```python
from build123d import *

# Parameters (mm, degrees)
SKETCH1_R           = 27
SKETCH1_R_2         = 1
SKETCH1_W           = 2
SKETCH1_H           = 6
SKETCH1_W_2         = 6
SKETCH1_H_2         = 2
BOSS_EXTRUDE1_DEPTH = 2


with BuildPart() as part:
    # Sketch1 → Boss-Extrude1 (new body)
    with BuildSketch(Plane.XY):
        with BuildLine():
            Line((23, 35), (35, 23))
            Line((35, 23), (35, 19))
            ThreePointArc((35, 19), (31, 0), (35, -19))
            Line((35, -19), (35, -23))
            Line((35, -23), (23, -35))
            Line((23, -35), (19, -35))
            ThreePointArc((19, -35), (0, -31), (-19, -35))
            Line((-19, -35), (-23, -35))
            Line((-23, -35), (-35, -23))
            Line((-35, -23), (-35, -19))
            ThreePointArc((-35, -19), (-31, 0), (-35, 19))
            Line((-35, 19), (-35, 23))
            Line((-35, 23), (-23, 35))
            Line((-23, 35), (-19, 35))
            ThreePointArc((-19, 35), (0, 31), (19, 35))
            Line((19, 35), (23, 35))
        make_face()
        Circle(SKETCH1_R, mode=Mode.SUBTRACT)
        with Locations((26, 26)):
            Circle(SKETCH1_R_2, mode=Mode.SUBTRACT)
        with Locations((21, 21)):
            Circle(SKETCH1_R_2, mode=Mode.SUBTRACT)
        with Locations((26, -26)):
            Circle(SKETCH1_R_2, mode=Mode.SUBTRACT)
        with Locations((-26, -26)):
            Circle(SKETCH1_R_2, mode=Mode.SUBTRACT)
        with Locations((-26, 26)):
            Circle(SKETCH1_R_2, mode=Mode.SUBTRACT)
        with BuildLine():
            Line((18, 30.970831308), (18, 24.718414189))
            ThreePointArc((18, 24.718414189), (17.465474668, 23.833352985), (16.433333333, 23.894467049))
            ThreePointArc((16.433333333, 23.894467049), (12.522883391, 26.15678481), (8.308523463, 27.78432))
            ThreePointArc((8.308523463, 27.78432), (7.59677162, 28.801490124), (8.423552466, 29.727589027))
            ThreePointArc((8.423552466, 29.727589027), (12.589647358, 30.640619364), (16.66084788, 31.911562853))
            ThreePointArc((16.66084788, 31.911562853), (17.574825139, 31.789107582), (18, 30.970831308))
        make_face(mode=Mode.SUBTRACT)
        with BuildLine():
            Line((-18, 30.970831308), (-18, 24.718414189))
            ThreePointArc((-18, 24.718414189), (-17.465474668, 23.833352985), (-16.433333333, 23.894467049))
            ThreePointArc((-16.433333333, 23.894467049), (-12.522883391, 26.156784809), (-8.308523463, 27.78432))
            ThreePointArc((-8.308523463, 27.78432), (-7.59677162, 28.801490124), (-8.423552466, 29.727589027))
            ThreePointArc((-8.423552466, 29.727589027), (-12.589647358, 30.640619364), (-16.66084788, 31.911562853))
            ThreePointArc((-16.66084788, 31.911562853), (-17.574825139, 31.789107582), (-18, 30.970831308))
        make_face(mode=Mode.SUBTRACT)
        with Locations((-21, 29)):
            Rectangle(SKETCH1_W, SKETCH1_H, mode=Mode.SUBTRACT)
        with Locations((21, 29)):
            Rectangle(SKETCH1_W, SKETCH1_H, mode=Mode.SUBTRACT)
        with Locations((29, 21)):
            Rectangle(SKETCH1_W_2, SKETCH1_H_2, mode=Mode.SUBTRACT)
        with Locations((29, -21)):
            Rectangle(SKETCH1_W_2, SKETCH1_H_2, mode=Mode.SUBTRACT)
        with BuildLine():
            Line((30.970831308, 18), (24.718414189, 18))
            ThreePointArc((24.718414189, 18), (23.833352985, 17.465474668), (23.894467049, 16.433333333))
            ThreePointArc((23.894467049, 16.433333333), (26.156784809, 12.522883391), (27.78432, 8.308523463))
            ThreePointArc((27.78432, 8.308523463), (28.801490124, 7.59677162), (29.727589027, 8.423552466))
            ThreePointArc((29.727589027, 8.423552466), (30.640619364, 12.589647358), (31.911562853, 16.66084788))
            ThreePointArc((31.911562853, 16.66084788), (31.789107582, 17.574825139), (30.970831308, 18))
        make_face(mode=Mode.SUBTRACT)
        with BuildLine():
            Line((30.970831308, -18), (24.718414189, -18))
            ThreePointArc((24.718414189, -18), (23.833352985, -17.465474668), (23.894467049, -16.433333333))
            ThreePointArc((23.894467049, -16.433333333), (26.15678481, -12.522883391), (27.78432, -8.308523463))
            ThreePointArc((27.78432, -8.308523463), (28.801490124, -7.59677162), (29.727589027, -8.423552466))
            ThreePointArc((29.727589027, -8.423552466), (30.640619364, -12.589647358), (31.911562853, -16.66084788))
            ThreePointArc((31.911562853, -16.66084788), (31.789107582, -17.574825139), (30.970831308, -18))
        make_face(mode=Mode.SUBTRACT)
        with Locations((21, -29)):
            Rectangle(SKETCH1_W, SKETCH1_H, mode=Mode.SUBTRACT)
        with Locations((-21, -29)):
            Rectangle(SKETCH1_W, SKETCH1_H, mode=Mode.SUBTRACT)
        with BuildLine():
            Line((18, -30.970831308), (18, -24.718414189))
            ThreePointArc((18, -24.718414189), (17.465474668, -23.833352985), (16.433333333, -23.894467049))
            ThreePointArc((16.433333333, -23.894467049), (12.522883391, -26.156784809), (8.308523463, -27.78432))
            ThreePointArc((8.308523463, -27.78432), (7.59677162, -28.801490124), (8.423552466, -29.727589027))
            ThreePointArc((8.423552466, -29.727589027), (12.589647358, -30.640619364), (16.66084788, -31.911562853))
            ThreePointArc((16.66084788, -31.911562853), (17.574825139, -31.789107582), (18, -30.970831308))
        make_face(mode=Mode.SUBTRACT)
        with BuildLine():
            Line((-18, -30.970831308), (-18, -24.718414189))
            ThreePointArc((-18, -24.718414189), (-17.465474668, -23.833352985), (-16.433333333, -23.894467049))
            ThreePointArc((-16.433333333, -23.894467049), (-12.522883391, -26.15678481), (-8.308523463, -27.78432))
            ThreePointArc((-8.308523463, -27.78432), (-7.59677162, -28.801490124), (-8.423552466, -29.727589027))
            ThreePointArc((-8.423552466, -29.727589027), (-12.589647358, -30.640619364), (-16.66084788, -31.911562853))
            ThreePointArc((-16.66084788, -31.911562853), (-17.574825139, -31.789107582), (-18, -30.970831308))
        make_face(mode=Mode.SUBTRACT)
        with Locations((-29, -21)):
            Rectangle(SKETCH1_W_2, SKETCH1_H_2, mode=Mode.SUBTRACT)
        with Locations((-29, 21)):
            Rectangle(SKETCH1_W_2, SKETCH1_H_2, mode=Mode.SUBTRACT)
        with BuildLine():
            Line((-30.970831308, -18), (-24.718414189, -18))
            ThreePointArc((-24.718414189, -18), (-23.833352985, -17.465474668), (-23.894467049, -16.433333333))
            ThreePointArc((-23.894467049, -16.433333333), (-26.156784809, -12.522883391), (-27.78432, -8.308523463))
            ThreePointArc((-27.78432, -8.308523463), (-28.801490124, -7.59677162), (-29.727589027, -8.423552466))
            ThreePointArc((-29.727589027, -8.423552466), (-30.640619364, -12.589647358), (-31.911562853, -16.66084788))
            ThreePointArc((-31.911562853, -16.66084788), (-31.789107582, -17.574825139), (-30.970831308, -18))
        make_face(mode=Mode.SUBTRACT)
        with BuildLine():
            Line((-30.970831308, 18), (-24.718414189, 18))
            ThreePointArc((-24.718414189, 18), (-23.833352985, 17.465474668), (-23.894467049, 16.433333333))
            ThreePointArc((-23.894467049, 16.433333333), (-26.15678481, 12.522883391), (-27.78432, 8.308523463))
            ThreePointArc((-27.78432, 8.308523463), (-28.801490124, 7.59677162), (-29.727589027, 8.423552466))
            ThreePointArc((-29.727589027, 8.423552466), (-30.640619364, 12.589647358), (-31.911562853, 16.66084788))
            ThreePointArc((-31.911562853, 16.66084788), (-31.789107582, 17.574825139), (-30.970831308, 18))
        make_face(mode=Mode.SUBTRACT)
    extrude(amount=BOSS_EXTRUDE1_DEPTH)


solid = part.part
```
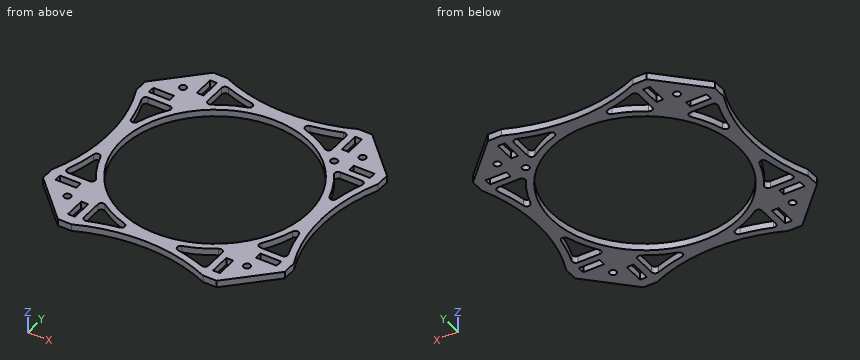
Part model, mm, in its own coordinate system. Round coordinates to 2 decimals unless told otherwise and drop trailing zeros. Order: outer loops, then holes, each group sorted by start corner. A loop starts at its lowest first (then second) coordinate and runs counter-clockwise, first axis right, second up. Notation, with made-up numbers: M 4,72.5 L 39,72.5 A23 ccw 39,109.5 Z; hole C 55.25,-34.75 d1. An arc over 180 degrees is marked long. Answer in a Markdown table with one row per item. Add a question column.
Q1. Wall check: L1, parallel to X at y = -29, z = 1.65; L2, parallel to X at y = -1, z = 1.6; L3, parallel to X at y = -11, z = 0.95. Give the ranges that are in metal, low to high. Write a range as from..to.
Q2. Cut at A-A on x = 0. Give the cut face in (y, z).
Q3. Pin check, flat tips, straight feed: pin 1 (0.6 mm diameter, centred on y = 29.5, z = 0.5, fed in from -X); pin 2 (0.6 mm diameter, centred on y = -28, z = 1, fed in from +X); pin 3 (0.6 mm diameter, centred on x = -29.5, z = 1.5, fed in from -Y); pin 4 (12 mm diameter, centred on x = 15.5, y = 11, fed in from +Z). Stop position of each tip, or through.
Q4. Cut at C-C on x = 21. Give the cut face in (y, z).
Established:
| question | item | result |
|---|---|---|
| 1 | L1 | x = -29..-22, -20..-18, -7.63..7.63, 18..20, 22..29 |
| 1 | L2 | x = -31.01..-26.98, 26.98..31.01 |
| 1 | L3 | x = -32.3..-30.25, -26.83..-24.66, 24.66..26.83, 30.25..32.3 |
| 2 | outline | M -31,0 L -27,0 L -27,2 L -31,2 Z; M 27,0 L 31,0 L 31,2 L 27,2 Z |
| 3 | pin 1 | stops at x = -28.8 |
| 3 | pin 2 | stops at x = 30.3 |
| 3 | pin 3 | stops at y = -28.8 |
| 3 | pin 4 | passes through |
| 4 | outline | M -35,0 L -32,0 L -32,2 L -35,2 Z; M -26,0 L -16.97,0 L -16.97,2 L -26,2 Z; M 16.97,0 L 20,0 L 20,2 L 16.97,2 Z; M 22,0 L 26,0 L 26,2 L 22,2 Z; M 32,0 L 35,0 L 35,2 L 32,2 Z |
